For this review, take the finished solid that the model builds, in its own axes (mm). A direction names the side the tool comes from. Give positions to 0.01 mm unless a question says otherwise; leave off trailing zeros. Write each loop counter-clockwise with the first axis right and the second up, starting at its lowest first coordinate (ties: lowest second). Pieces come first, ordered by that corner, then holes.
Q1. We need section B-B (x = 9). Write out the cut boundary in (y, z), then the cut area to 3 significant figures.
Q2. Mouldability with a two-part tool opening along Z and no side actions: class faces 3 (the cylindrical face through (17.68, 0.789, -6.227)), 4 (the cylindrical face through (14.9, 0.79, -11.98)), 5 (the cylindrical face through (-22.5, 0.8, -0.2)), 6 (the cylindrical face through (14.851, 0.789, 11.993)) as released by +Z, released by -Z, zero draft, split by the parting line, or undercut.
Q3. Machinability: for faces 1 (the cylindrical face through (-14.851, 0.789, -11.993)), 2 (the cylindrical face through (-17.68, 0.789, 6.227)), which of the approach directions +Z, -Z, +X, -X, +Y, -Y give a long, thin tool a straight path to every point of the face, cutting with its end or side? Answer none if there is none.
Q4. We need section A-A (z = -5.5). Write out the cut boundary in (x, y).
Q5. For line 1 (X direction, y = 0.4, z = -0.5); line 2 (Z direction, x = -7, y = 0.8); line 3 (X direction, y = 0.85, z = 10), list the stretches that pass through material, from the lowest coordinate up.
```python
from build123d import *

# Parameters (mm, degrees)
BOSS_EXTRUDE1_DEPTH = 1.6
CUT_EXTRUDE2_DEPTH  = 2.6


with BuildPart() as part:
    # Internal Slab → Boss-Extrude1 (new body)
    with BuildSketch(Plane(origin=(0, 0, 0), x_dir=(1, 0, 0), z_dir=(0, 1, 0))):
        with BuildLine():
            ThreePointArc((19.864398082, 10.566725549), (18.521398428, 11.814512636), (16.694380928, 11.964937844))
            ThreePointArc((16.694380928, 11.964937844), (14.875391632, 11.986370035), (13.312847331, 12.91784022))
            ThreePointArc((13.312847331, 12.91784022), (13.116830791, 13.116830791), (12.91784022, 13.312847331))
            ThreePointArc((12.91784022, 13.312847331), (11.986370035, 14.875391632), (11.964937844, 16.694380928))
            ThreePointArc((11.964937844, 16.694380928), (12.030759646, 17.039737643), (12.052815994, 17.390618375))
            ThreePointArc((12.052815994, 17.390618375), (11.652730082, 18.833536499), (10.566725549, 19.864398082))
            ThreePointArc((10.566725549, 19.864398082), (0, 22.5), (-10.566725549, 19.864398082))
            ThreePointArc((-10.566725549, 19.864398082), (-11.814512636, 18.521398428), (-11.964937844, 16.694380928))
            ThreePointArc((-11.964937844, 16.694380928), (-11.986370035, 14.875391632), (-12.91784022, 13.312847331))
            ThreePointArc((-12.91784022, 13.312847331), (-13.116830791, 13.116830791), (-13.312847331, 12.91784022))
            ThreePointArc((-13.312847331, 12.91784022), (-14.875391632, 11.986370035), (-16.694380928, 11.964937844))
            ThreePointArc((-16.694380928, 11.964937844), (-17.039737643, 12.030759646), (-17.390618375, 12.052815994))
            ThreePointArc((-17.390618375, 12.052815994), (-18.833536499, 11.652730082), (-19.864398082, 10.566725549))
            ThreePointArc((-19.864398082, 10.566725549), (-22.5, 0), (-19.864398082, -10.566725549))
            ThreePointArc((-19.864398082, -10.566725549), (-18.521398428, -11.814512636), (-16.694380928, -11.964937844))
            ThreePointArc((-16.694380928, -11.964937844), (-14.875391632, -11.986370035), (-13.312847331, -12.91784022))
            ThreePointArc((-13.312847331, -12.91784022), (-13.116830791, -13.116830791), (-12.91784022, -13.312847331))
            ThreePointArc((-12.91784022, -13.312847331), (-11.986370035, -14.875391632), (-11.964937844, -16.694380928))
            ThreePointArc((-11.964937844, -16.694380928), (-12.030759646, -17.039737643), (-12.052815994, -17.390618375))
            ThreePointArc((-12.052815994, -17.390618375), (-11.652730082, -18.833536499), (-10.566725549, -19.864398082))
            ThreePointArc((-10.566725549, -19.864398082), (0, -22.5), (10.566725549, -19.864398082))
            ThreePointArc((10.566725549, -19.864398082), (11.814512636, -18.521398428), (11.964937844, -16.694380928))
            ThreePointArc((11.964937844, -16.694380928), (11.986370035, -14.875391632), (12.91784022, -13.312847331))
            ThreePointArc((12.91784022, -13.312847331), (13.116830791, -13.116830791), (13.312847331, -12.91784022))
            ThreePointArc((13.312847331, -12.91784022), (14.875391632, -11.986370035), (16.694380928, -11.964937844))
            ThreePointArc((16.694380928, -11.964937844), (17.039737643, -12.030759646), (17.390618375, -12.052815994))
            ThreePointArc((17.390618375, -12.052815994), (18.833536499, -11.652730082), (19.864398082, -10.566725549))
            ThreePointArc((19.864398082, -10.566725549), (22.5, 0), (19.864398082, 10.566725549))
        make_face()
    extrude(amount=BOSS_EXTRUDE1_DEPTH)

    # Sketch3 → Cut-Extrude2 (cut, through all)
    with BuildSketch(Plane(origin=(0, 0, 0), x_dir=(1, 0, 0), z_dir=(0, 1, 0))):
        with BuildLine():
            ThreePointArc((-14.443108961, 7.983520749), (-17.643874139, 6.264479657), (-19.265757154, 3.013403606))
            ThreePointArc((-19.265757154, 3.013403606), (-19.441351091, 1.511247085), (-19.5, 0))
            ThreePointArc((-19.5, 0), (-19.441351091, -1.511247085), (-19.265757154, -3.013403606))
            ThreePointArc((-19.265757154, -3.013403606), (-17.643874139, -6.264479657), (-14.443108961, -7.983520749))
            ThreePointArc((-14.443108961, -7.983520749), (-12.276076656, -8.747806411), (-10.442152488, -10.132322113))
            ThreePointArc((-10.442152488, -10.132322113), (-10.288403666, -10.288403666), (-10.132322113, -10.442152488))
            ThreePointArc((-10.132322113, -10.442152488), (-8.747806411, -12.276076656), (-7.983520749, -14.443108961))
            ThreePointArc((-7.983520749, -14.443108961), (-6.264479657, -17.643874139), (-3.013403606, -19.265757154))
            ThreePointArc((-3.013403606, -19.265757154), (-1.511247085, -19.441351091), (0, -19.5))
            ThreePointArc((0, -19.5), (1.511247085, -19.441351091), (3.013403606, -19.265757154))
            ThreePointArc((3.013403606, -19.265757154), (6.264479657, -17.643874139), (7.983520749, -14.443108961))
            ThreePointArc((7.983520749, -14.443108961), (8.747806411, -12.276076656), (10.132322113, -10.442152488))
            ThreePointArc((10.132322113, -10.442152488), (10.288403666, -10.288403666), (10.442152488, -10.132322113))
            ThreePointArc((10.442152488, -10.132322113), (12.276076656, -8.747806411), (14.443108961, -7.983520749))
            ThreePointArc((14.443108961, -7.983520749), (17.643874139, -6.264479657), (19.265757154, -3.013403606))
            ThreePointArc((19.265757154, -3.013403606), (19.441351091, -1.511247085), (19.5, 0))
            ThreePointArc((19.5, 0), (19.441351091, 1.511247085), (19.265757154, 3.013403606))
            ThreePointArc((19.265757154, 3.013403606), (17.643874139, 6.264479657), (14.443108961, 7.983520749))
            ThreePointArc((14.443108961, 7.983520749), (12.276076656, 8.747806411), (10.442152488, 10.132322113))
            ThreePointArc((10.442152488, 10.132322113), (10.288403666, 10.288403666), (10.132322113, 10.442152488))
            ThreePointArc((10.132322113, 10.442152488), (8.747806411, 12.276076656), (7.983520749, 14.443108961))
            ThreePointArc((7.983520749, 14.443108961), (6.264479657, 17.643874139), (3.013403606, 19.265757154))
            ThreePointArc((3.013403606, 19.265757154), (1.511247085, 19.441351091), (0, 19.5))
            ThreePointArc((0, 19.5), (-1.511247085, 19.441351091), (-3.013403606, 19.265757154))
            ThreePointArc((-3.013403606, 19.265757154), (-6.264479657, 17.643874139), (-7.983520749, 14.443108961))
            ThreePointArc((-7.983520749, 14.443108961), (-8.747806411, 12.276076656), (-10.132322113, 10.442152488))
            ThreePointArc((-10.132322113, 10.442152488), (-10.288403666, 10.288403666), (-10.442152488, 10.132322113))
            ThreePointArc((-10.442152488, 10.132322113), (-12.276076656, 8.747806411), (-14.443108961, 7.983520749))
        make_face()
    extrude(amount=CUT_EXTRUDE2_DEPTH, mode=Mode.SUBTRACT)


solid = part.part
```
Computed:
1. outline: (0, -20.62) - (1.6, -20.62) - (1.6, -11.84) - (0, -11.84) - close; (0, 11.84) - (1.6, 11.84) - (1.6, 20.62) - (0, 20.62) - close
1. area: 28.1 mm2
2. face 3: undercut
2. face 4: released by -Z
2. face 5: split by the parting line
2. face 6: released by +Z
3. face 1: -Z, +Y, -Y
3. face 2: +Y, -Y
4. outline: (-21.82, 0) - (-18.27, 0) - (-18.27, 1.6) - (-21.82, 1.6) - close; (18.27, 0) - (21.82, 0) - (21.82, 1.6) - (18.27, 1.6) - close
5. line 1: x = -22.49 to -19.49, 19.49 to 22.49
5. line 2: z = -21.38 to -16.78, 16.78 to 21.38
5. line 3: x = -20.16 to -10.57, 10.57 to 20.16
